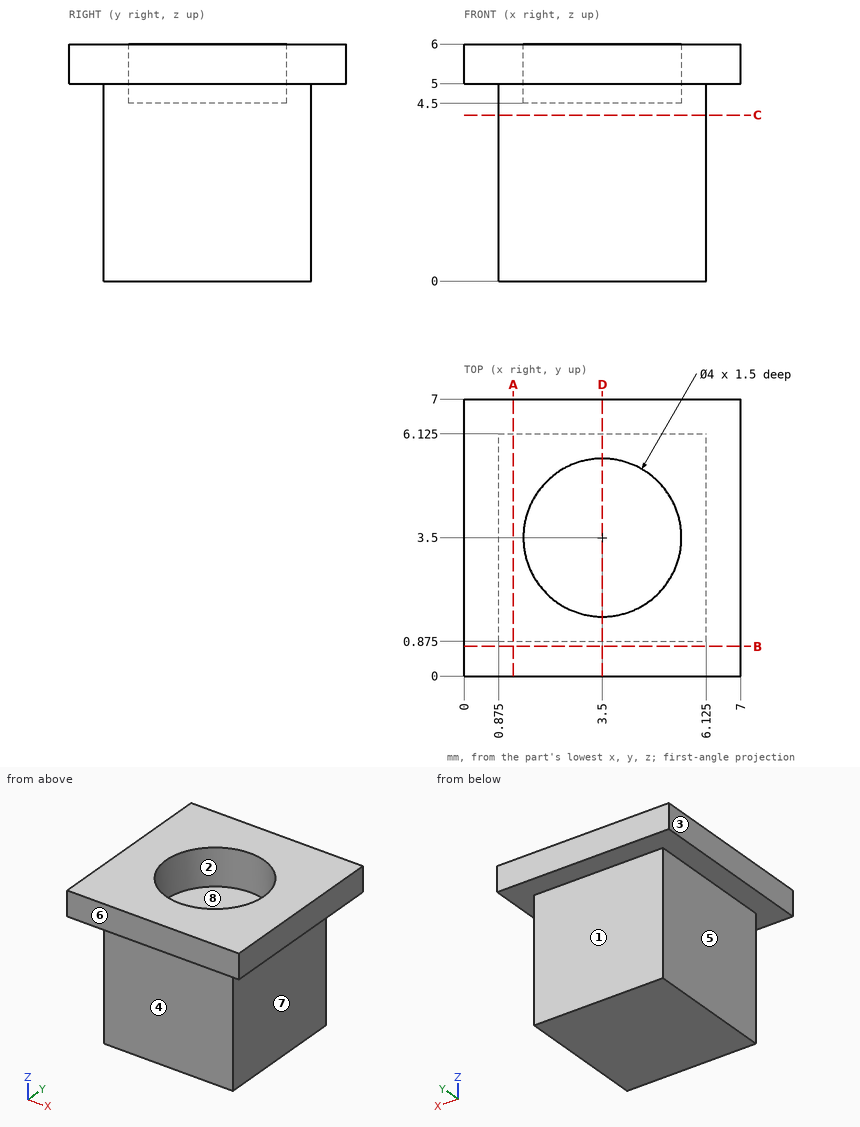
Can you work these out from the drawing? Everything is in mm from the part's minimum corner. A direction names the side the tool comes from. Round coordinates to 2 decimals unless told otherwise and drop trailing zeros. Order: outer loops, then holes, each group sorted by start corner. A loop starts at its lowest first (then second) coordinate and runs counter-clockwise, first axis right, second up.
(1) If we section it at A-A (x = 1.25): Please give me the cut outline in (y, z) (3 decimals).
Results are:
outline: (0, 5) - (0.875, 5) - (0.875, 0) - (6.125, 0) - (6.125, 5) - (7, 5) - (7, 6) - (0, 6) - close
(2) If we section it at C-C (z = 4.2): Please give me the cut outline in (x, y) (3 decimals).
Results are:
outline: (0.875, 0.875) - (6.125, 0.875) - (6.125, 6.125) - (0.875, 6.125) - close
(3) On a 3-axis mill with a long thin cutter (end or side, diameter ignored), from which of +Z, -Z, +X, -X, +Y, -Y can I reach the whole of each face in a straight line? I mean the marked faces 1, 2, 3, 4 and 5. Say none if no direction works.
Results are:
face 1: -Z, +X, -X, +Y
face 2: +Z
face 3: +Z, -Z, -X, +Y, -Y
face 4: -Z, +X, -X, -Y
face 5: -Z, -X, +Y, -Y
(4) If I drill on L1, parallel to Y at x = 3.5, z = 5.35; L2, parallel to Z at x = 3.25, y = 6.75; L3, parallel to Y at x = 1.5, z = 2.75 (3 decimals), over which ranges is the centre line in solid material (lowest first)?
Results are:
L1: y = 0 to 1.5, 5.5 to 7
L2: z = 5 to 6
L3: y = 0.875 to 6.125
(5) If we section it at D-D (x = 3.5): Please give me the cut outline in (y, z) (3 decimals).
Results are:
outline: (0, 5) - (0.875, 5) - (0.875, 0) - (6.125, 0) - (6.125, 5) - (7, 5) - (7, 6) - (5.5, 6) - (5.5, 4.5) - (1.5, 4.5) - (1.5, 6) - (0, 6) - close
(6) I'm going to push flat-ended pins straight in: pin 1 (1.5 mm diameter, centred on x = 4.5, z = 1.5, fed in from -Y) (3 decimals); pin 2 (1.5 mm diameter, centred on y = 3, z = 2.5, fed in from -X) (3 decimals); pin 3 (2.5 mm diameter, centred on x = 3.5, y = 3.5, fed in from +Z). Where does each tip first touch, or does it pass through?
Results are:
pin 1: stops at y = 0.875
pin 2: stops at x = 0.875
pin 3: stops at z = 4.5
(7) We'd pull the mould along X, two halves only. Please class the marked faces 6, 7 and 8: +X half, -X half, draft (parallel to the pull), parting line (faces both ways), or undercut.
Results are:
face 6: draft
face 7: +X half
face 8: undercut
(8) If we section it at B-B (y = 0.75): Please give me the cut outline in (x, z), plus the area to 3 significant figures.
Results are:
outline: (0, 5) - (7, 5) - (7, 6) - (0, 6) - close
area: 7.00 mm2
